```python
from build123d import *

# Parameters (mm, degrees)
BOSS_EXTRU_1_DEPTH           = 3.81
CORPS_D_PLACER_COPIER2_ANGLE = 180
BOSS_EXTRU_2_START           = -25.4
ESQUISSE4_R                  = 9.5
BOSS_EXTRU_2_DEPTH           = 146.05
R_P_TITION_LIN_AIRE2_COUNT   = 3
R_P_TITION_LIN_AIRE2_PITCH   = 146.05
CORPS_D_PLACER_COPIER3_ANGLE = 120
CORPS_D_PLACER_COPIER4_ANGLE = 120
ESQUISSE5_R                  = 9.5
BOSS_EXTRU_3_DEPTH           = 27.94


with BuildPart() as part:
    # Esquisse1 → Boss.-Extru.1 (new body, symmetric)
    with BuildSketch(Plane.XY):
        with BuildLine():
            Line((-5.499261314, 15.875), (-10.998522628, 6.35))
            ThreePointArc((-10.998522628, 6.35), (0, -12.7), (10.998522628, 6.35))
            Line((10.998522628, 6.35), (5.499261314, 15.875))
            ThreePointArc((5.499261314, 15.875), (0, 19.05), (-5.499261314, 15.875))
        make_face()
    extrude(amount=BOSS_EXTRU_1_DEPTH, both=True)


with BuildPart() as body_2:
    # Corps-D_placer_Copier1: copy of part
    add(part.part.moved(Location((0, 0, 60.96))))


with BuildPart() as body_2_1:
    # Corps-D_placer_Copier2: moved
    add(body_2.part.rotate(Axis((0, 0, 0), (0, 0, 1)), CORPS_D_PLACER_COPIER2_ANGLE))


with BuildPart() as part_1:
    add(part.part)

    add(body_2_1.part)  # Boss.-Extru.2 merges body 2
    # Esquisse4 → Boss.-Extru.2 (add)
    with BuildSketch(Plane.XY.offset(BOSS_EXTRU_2_START)):
        Circle(ESQUISSE4_R)
    extrude(amount=BOSS_EXTRU_2_DEPTH)


with BuildPart() as r_p_tition_lin_aire2_1:
    # R_p_tition lin_aire2: pattern copy
    add(part_1.part.moved(Location(Vector(0, 0, 1) * (1 * R_P_TITION_LIN_AIRE2_PITCH))))


with BuildPart() as r_p_tition_lin_aire2_2:
    # R_p_tition lin_aire2: pattern copy
    add(part_1.part.moved(Location(Vector(0, 0, 1) * (2 * R_P_TITION_LIN_AIRE2_PITCH))))


with BuildPart() as r_p_tition_lin_aire2_1_1:
    # Corps-D_placer_Copier3: moved
    add(r_p_tition_lin_aire2_1.part.rotate(Axis((0, 0, 0), (0, 0, 1)), CORPS_D_PLACER_COPIER3_ANGLE))


with BuildPart() as r_p_tition_lin_aire2_2_1:
    # Corps-D_placer_Copier4: moved
    add(r_p_tition_lin_aire2_2.part.rotate(Axis((0, 0, 0), (0, 0, -1)), CORPS_D_PLACER_COPIER4_ANGLE))


with BuildPart() as part_2:
    add(part_1.part)

    # Esquisse5 → Boss.-Extru.3 (add)
    with BuildSketch(Plane(origin=(0, 0, -25.4), x_dir=(-1, 0, 0), z_dir=(0, 0, -1))):
        Circle(ESQUISSE5_R)
    extrude(amount=BOSS_EXTRU_3_DEPTH)


with BuildPart() as r_p_tition_lin_aire2_2_2:
    add(r_p_tition_lin_aire2_2_1.part)

    # Combiner1: union R_p_tition lin_aire2_1, part
    add(r_p_tition_lin_aire2_1_1.part)
    add(part_2.part)


solid = r_p_tition_lin_aire2_2_2.part
```
Geometry check sheet. Reference: the model listing, model coordinates, mm. A direction names the side the tool comes from. Round coordinates to 2 decimals unless told otherwise and drop trailing zeros. Loops run counter-clockwise (first coordinate to the right, second up) from the corner with the lowest first, then second, coordinate; pieces in that order, holes last. Notation, with made-up numbers: (-11, 37.5) -> (1, 37.5) arc R26 cw to (1, 69.5) -> close; hole circle Ø8 at (41, 8). An arc over 180 degrees is marked (long way). Use a Markdown table: item, result.
(1) Scan lines: probe 1 along Z at (x, y) = (-5.5, 11); probe 2 along Y at (x, z) = (-1, 377.5); probe 3 along Z at (x, y) = (-5.5, -13). Record each from-to range of solid material in increasing order.
Calculated:
| item | result |
|---|---|
| probe 1 | -3.81 to 3.81, 57.15 to 64.77, 142.24 to 149.86, 203.2 to 210.82, 288.29 to 295.91, 349.25 to 356.87 |
| probe 2 | -9.45 to 9.45 |
| probe 3 | 57.15 to 64.77 |
(2) Go/stop test with flat-tipped pins: P1, Ø5, axis at y = 9, z = 282.5, coming from the +X side; P2, Ø8, axis at x = -10, y = 11, coming from the +Z side; P3, Ø8.5, axis at x = -8, z = 353.5, coming from the +Y side; P4, Ø1.5, axis at y = -15, z = 211.5, coming from the -X side. Record where each tip stops, or that it passes through.
Calculated:
| item | result |
|---|---|
| P1 | x = 6.93 |
| P2 | z = 356.87 |
| P3 | y = 12.7 |
| P4 | through |
(3) Sectioned sample at A-A (z = 191). Enter the section's corners in (x, y), then the cut area to 3 significant figures.
Calculated:
| item | result |
|---|---|
| outline | circle Ø19 at (0, 0) |
| area | 284 mm² |
(4) Set-up check for faces 4 (the flat face through (13.71, -1.65, 207.06)), 5 (the cylindrical face through (10.808, -6.67, 353.113)), 6 (the cylindrical face through (0.372, 12.695, 61.013)): record each of +Z, -Z, +X, -X, +Y, -Y from which the full face is reachable in a straight line by a thin tool's end or side.
Calculated:
| item | result |
|---|---|
| face 4 | -Z, +X, -Y |
| face 5 | +Z |
| face 6 | none |
(5) Mould release check, pull along Z, two halves, no side actions. Record for faces 1 (the flat face through (-7, 7, 349.25)), 2 (the flat face through (0, 0, -53.34)), 3 (the flat face through (-6, -12.7, 146)): released by +Z, released by -Z, zero draft, split by the parting line, or undercut.
Calculated:
| item | result |
|---|---|
| face 1 | undercut |
| face 2 | released by -Z |
| face 3 | zero draft |
